Geometry check sheet. Reference: the model listing, model coordinates, mm. A direction names the side the tool comes from. Give positions to 0.01 mm unless a question says otherwise; leave off trailing zeros. Loops run counter-clockwise (first coordinate to the right, second up) from the corner with the lowest first, then second, coordinate; pieces in that order, holes last.
```python
from build123d import *

# Parameters (mm, degrees)
SKETCH1_R            = 10
BOSS_EXTRUDE1_DEPTH  = 20
SKETCH2_R            = 15
BOSS_EXTRUDE2_DEPTH  = 145
BOSS_EXTRUDE3_DEPTH  = 22
SKETCH4_R            = 11.540024106
BOSS_EXTRUDE4_DEPTH  = 20
BOSS_EXTRUDE7_DEPTH  = 25
SKETCH6_R            = 10
BOSS_EXTRUDE8_DEPTH  = 35
BOSS_EXTRUDE11_DEPTH = 22
SKETCH8_R            = 12.5
BOSS_EXTRUDE12_DEPTH = 22.5
SKETCH9_R            = 50
SKETCH9_R_2          = 5
BOSS_EXTRUDE13_DEPTH = 16


with BuildPart() as part:
    # Sketch1 → Boss-Extrude1 (new body)
    with BuildSketch(Plane(origin=(0, 0, 0), x_dir=(0, 0, -1), z_dir=(1, 0, 0))):
        Circle(SKETCH1_R)
    extrude(amount=-BOSS_EXTRUDE1_DEPTH)

    # Sketch2 → Boss-Extrude2 (add)
    with BuildSketch(Plane.ZY.offset(20)):
        Circle(SKETCH2_R)
    boss_extrude2 = extrude(amount=BOSS_EXTRUDE2_DEPTH)

    # Sketch3 → Boss-Extrude3 (add)
    with BuildSketch(Plane.ZY.offset(165)):
        with BuildLine():
            Line((-17.5, 40), (-17.5, 0))
            ThreePointArc((-17.5, 0), (0, -17.5), (17.5, 0))
            Line((17.5, 0), (17.5, 40))
            ThreePointArc((17.5, 40), (0, 57.5), (-17.5, 40))
        make_face()
    boss_extrude3 = extrude(amount=BOSS_EXTRUDE3_DEPTH)

    # Sketch4 → Boss-Extrude4 (add)
    with BuildSketch(Plane.ZY.offset(187)):
        with Locations((0, 40)):
            Circle(SKETCH4_R)
    boss_extrude4 = extrude(amount=BOSS_EXTRUDE4_DEPTH)

    # Sketch5 → Boss-Extrude7 (add)
    with BuildSketch(Plane.ZY.offset(207)):
        with BuildLine():
            Line((-17.5, 40), (-17.5, -30))
            ThreePointArc((-17.5, -30), (0, -47.5), (17.5, -30))
            Line((17.5, -30), (17.5, 40))
            ThreePointArc((17.5, 40), (0, 57.5), (-17.5, 40))
        make_face()
    boss_extrude7 = extrude(amount=BOSS_EXTRUDE7_DEPTH)

    # Sketch6 → Boss-Extrude8 (add)
    with BuildSketch(Plane.ZY.offset(232)):
        with Locations((0, -30)):
            Circle(SKETCH6_R)
    boss_extrude8 = extrude(amount=BOSS_EXTRUDE8_DEPTH)

    # Sketch7 → Boss-Extrude11 (add)
    with BuildSketch(Plane.ZY.offset(267)):
        with BuildLine():
            Line((17.499097446, 14.822268204), (17.5, -30))
            ThreePointArc((17.5, -30), (0, -47.5), (-17.5, -30))
            Line((-17.5, -30), (-17.5, 15))
            ThreePointArc((-17.5, 15), (0.088867044, 32.49977436), (17.499097446, 14.822268204))
        make_face()
    boss_extrude11 = extrude(amount=BOSS_EXTRUDE11_DEPTH)

    # Sketch8 → Boss-Extrude12 (add)
    with BuildSketch(Plane.ZY.offset(289)):
        with Locations(Location((0, 15, 0), (0, 0, 180))):
            Circle(SKETCH8_R)
    boss_extrude12 = extrude(amount=BOSS_EXTRUDE12_DEPTH)

    # Mirror5: Boss-Extrude12 across plane
    add(boss_extrude12.mirror(Plane(origin=(-311.5, 15, 0), x_dir=(0, 0, 1), z_dir=(-1, 0, 0))))

    # Mirror6: Boss-Extrude11 across plane
    add(boss_extrude11.mirror(Plane.ZY.offset(311.5)))

    # Mirror7: Boss-Extrude8 across plane
    add(boss_extrude8.mirror(Plane.ZY.offset(311.5)))

    # Mirror8: Boss-Extrude7 across plane
    add(boss_extrude7.mirror(Plane.ZY.offset(311.5)))

    # Mirror9: Boss-Extrude4 across plane
    add(boss_extrude4.mirror(Plane.ZY.offset(311.5)))

    # Mirror10: Boss-Extrude3 across plane
    add(boss_extrude3.mirror(Plane.ZY.offset(311.5)))

    # Mirror11: Boss-Extrude2 across plane
    add(boss_extrude2.mirror(Plane.ZY.offset(311.5)))

    # Sketch9 → Boss-Extrude13 (add)
    with BuildSketch(Plane.ZY.offset(603)):
        Circle(SKETCH9_R)
        with Locations((0, 27.436873089)):
            Circle(SKETCH9_R_2, mode=Mode.SUBTRACT)
        with Locations((27.436873089, 0)):
            Circle(SKETCH9_R_2, mode=Mode.SUBTRACT)
        with Locations((0, -27.436873089)):
            Circle(SKETCH9_R_2, mode=Mode.SUBTRACT)
        with Locations((-27.436873089, 0)):
            Circle(SKETCH9_R_2, mode=Mode.SUBTRACT)
    extrude(amount=BOSS_EXTRUDE13_DEPTH)


solid = part.part
```
1) Sectioned sample at C-C on x = -141. Enter the section's corners in (y, z).
2) Sectioned sample at A-A on x = -239. Enter the section's corners in (y, z), plus the area to 3 significant figures.
3) Tool access check on faces 1 (the flat face through (-176, 20, 17.5)), 2 (the flat face through (-345, -8, -17.5)), 3 (the cylindrical face through (-403.675, -47.496, -0.385)). Record the directions out of +Z, -Z, +X, -X, +Y, -Y that give a thin tool (end or side, any length) a straight path to the whole face; none if there is none.
4) Sectioned sample at B-B on z = -38.5. Enter the section's corners in (x, y), plus the area to 3 significant figures.
5) Mould release check, pull along X, two halves, no side actions. Record for faces 4 (the flat face through (-356, -7, 0)), 5 (the cylindrical face through (-610.888, 1.502, -22.668)), 6 (the flat face through (-334, -16, 0)), 7 (the flat face through (-20, -10, 3)): +X half, -X half, draft (parallel to the pull), parting line (faces both ways), or undercut.
6) Depth check by flat-ended pin: P1, Ø17.5, axis at y = 28.5, z = -2.5, coming from the +X side; P2, Ø11, axis at x = -344.5, y = 1, coming from the -Z side; P3, Ø6.5, axis at x = -173, y = 12, coming from the +Z side. Enter the tip coordinate at first touch or a pass-through.
7) Scan lines: line 1 along X through (y, z) = (-6, -0.5); line 2 along X through (y, z) = (23.5, 1.5); line 3 along X through (y, z) = (40.5, 2.5). Record each from-to range of solid material in increasing order.
8) Sectioned sample at D-D on x = -344. Enter the section's corners in (y, z), plus the area to 3 significant figures.
Determined:
1. outline: circle Ø30 at (0, 0)
2. outline: circle Ø20 at (-30, 0)
2. area: 314 mm2
3. face 1: +Z, +X, +Y, -Y
3. face 2: -Z, +X, +Y, -Y
3. face 3: +X, -Y
4. outline: (-619, -31.9) - (-603, -31.9) - (-603, 31.9) - (-619, 31.9) - close
4. area: 1,020 mm2
5. face 4: undercut
5. face 5: draft
5. face 6: undercut
5. face 7: +X half
6. P1: stops at x = -165
6. P2: stops at z = -17.5
6. P3: stops at z = 17.5
7. line 1: x = -619 to -436, -416 to -391, -356 to -334, -289 to -267, -232 to -207, -187 to 0
7. line 2: x = -458 to -436, -416 to -391, -356 to -267, -232 to -207, -187 to -165
7. line 3: x = -619 to -603, -458 to -391, -232 to -165
8. outline: (-30, -17.5) - (15, -17.5) arc R17.5 ccw (long way) to (14.82, 17.5) - (-30, 17.5) arc R17.5 ccw to start
8. area: 2,540 mm2
